```python
from build123d import *

# Parameters (mm, degrees)
F0_W      = 30.1625
F0_H      = 6.35
F1_DEPTH  = 26.9875
F3_DEPTH  = 6.351
F4_W      = 12.7
F4_H      = 6.35
F5_DEPTH  = 6.351
F6_W      = 6.35
F6_H      = 1.5875
F7_DEPTH  = 7.9375
F8_W      = 12.7
F8_H      = 6.35
F9_DEPTH  = 3
F10_W     = 12.7
F10_H     = 6.35
F11_DEPTH = 3
F12_W     = 6.35
F12_H     = 10.9375
F13_DEPTH = 8
F14_W     = 6.35
F14_H     = 9.35
F15_DEPTH = 8
F16_W     = 6.35
F16_H     = 17.6375
F17_DEPTH = 1
F18_W     = 6.35
F18_H     = 11.2875
F19_DEPTH = 1
F20_W     = 24.8125
F20_H     = 6.35
F21_DEPTH = 1
F22_W     = 31.1625
F22_H     = 6.35
F23_DEPTH = 1


with BuildPart() as f1:
    # F0 (on Top) → F1 (new body)
    with BuildSketch(Plane.XY):
        with Locations((3.826838, -2.493716)):
            Rectangle(F0_W, F0_H)
    extrude(amount=F1_DEPTH)

    # F2 (on face) → F3 (cut, through all)
    with BuildSketch(Plane.XZ.offset(5.668716)):
        Polygon((15.733088, 9.525), (15.733088, 23.8125), (-8.079412, 23.8125), (-8.079412, 1.5875), (-4.904412, 1.5875), (-4.904412, 0), (3.033088, 0), (3.033088, 9.525), align=None)
    extrude(amount=-F3_DEPTH, mode=Mode.SUBTRACT)

    # F4 (on face) → F5 (cut, through all)
    with BuildSketch(Plane.XZ.offset(5.668716)):
        with Locations((12.558088, 3.175)):
            Rectangle(F4_W, F4_H)
    extrude(amount=-F5_DEPTH, mode=Mode.SUBTRACT)

    # F6 (on face) → F7 (join)
    with BuildSketch(Plane.YZ.offset(-4.904412)):
        with Locations((-2.493716, 0.79375)):
            Rectangle(F6_W, F6_H)
    extrude(amount=F7_DEPTH)

    # F8 (on face) → F9 (join)
    with BuildSketch(Plane.XY.offset(9.525)):
        with Locations((9.383088, -2.493716)):
            Rectangle(F8_W, F8_H)
    extrude(amount=F9_DEPTH)

    # F10 (on face) → F11 (cut)
    with BuildSketch(Plane(origin=(0, 0, 6.35), x_dir=(1, 0, 0), z_dir=(0, 0, -1))):
        with Locations((12.558088, 2.493716)):
            Rectangle(F10_W, F10_H)
    extrude(amount=-F11_DEPTH, mode=Mode.SUBTRACT)

    # F12 (on face) → F13 (join)
    with BuildSketch(Plane(origin=(3.033088, 0, 0), x_dir=(0, -1, 0), z_dir=(-1, 0, 0))):
        with Locations((2.493716, 7.05625)):
            Rectangle(F12_W, F12_H)
    extrude(amount=F13_DEPTH)

    # F14 (on face) → F15 (cut)
    with BuildSketch(Plane.YZ.offset(6.208088)):
        with Locations((-2.493716, 4.675)):
            Rectangle(F14_W, F14_H)
    extrude(amount=-F15_DEPTH, mode=Mode.SUBTRACT)

    # F16 (on face) → F17 (join)
    with BuildSketch(Plane.YZ.offset(18.908088)):
        with Locations((-2.493716, 18.16875)):
            Rectangle(F16_W, F16_H)
    extrude(amount=F17_DEPTH)

    # F18 (on face) → F19 (cut)
    with BuildSketch(Plane(origin=(15.733088, 0, 0), x_dir=(0, -1, 0), z_dir=(-1, 0, 0))):
        with Locations((2.493716, 18.16875)):
            Rectangle(F18_W, F18_H)
    extrude(amount=-F19_DEPTH, mode=Mode.SUBTRACT)

    # F20 (on face) → F21 (cut)
    with BuildSketch(Plane(origin=(0, 0, 23.8125), x_dir=(1, 0, 0), z_dir=(0, 0, -1))):
        with Locations((4.326838, 2.493716)):
            Rectangle(F20_W, F20_H)
    extrude(amount=-F21_DEPTH, mode=Mode.SUBTRACT)

    # F22 (on face) → F23 (join)
    with BuildSketch(Plane.XY.offset(26.9875)):
        with Locations((4.326838, -2.493716)):
            Rectangle(F22_W, F22_H)
    extrude(amount=F23_DEPTH)


solid = f1.part
```
Geometry check sheet. Reference: the model listing, model coordinates, mm. A direction names the side the tool comes from. Give positions to 0.01 mm unless a question says otherwise; leave off trailing zeros. Loops run counter-clockwise (first coordinate to the right, second up) from the corner with the lowest first, then second, coordinate; pieces in that order, holes last. Notation, with made-up numbers: (-22, 54) - (6, 54) arc R15 ccw to (6, 59) - close; hole circle Ø4 at (-30.5, 9). An arc over 180 degrees is marked (long way). Use CSV: the item, a comma, the result in double quotes. Start each with the question number.
Q1. Go/stop test with flat-tipped pins: pin 1 Ø3 at (x, y) = (6.5, -3) entering from -Z; pin 2 Ø4 at (x, z) = (-6, 20.5) entering from +Y; pin 3 Ø3 at (y, z) = (-3.5, 3) entering from +X. Record where each tip stops, or that it passes through.
Q2. Release check for a two-part mould opening along X. For faces 4 (the face through (-1.792, -3, 5)), 5 (the face through (6, -2, 12.525)), 6 (the face through (1, 0.681, 11)) record: +X half, -X half, draft (parallel to the pull), parting line (faces both ways), or undercut.
Q3. Access from +Z, -Z, +X, -X, +Y, -Y to the whole of each face (thin tool, end or side, straight path). Record for faces 1 (the face through (19.908, -3, 19)), 2 (the face through (-8.079, -2, 13)), 3 (the face through (9, -3, 9.35)).
Q4. Scan lines: probe 1 along X at (y, z) = (-4.75, 14.75); probe 2 along X at (y, z) = (-2.5, 6); probe 3 along Z at (x, y) = (-2, -1.25) (1 decimal). Record each from-to range of solid material in increasing order. Write a range as from..to.
Q5. Section check A-A, the plane z = 9.75. Record the cut outline in (x, y).
Findings below:
1,pin 1,"stops at z = 9.35"
1,pin 2,"passes through"
1,pin 3,"stops at x = -1.79"
2,face 4,"+X half"
2,face 5,"undercut"
2,face 6,"draft"
3,face 1,"+Z, -Z, +X, +Y, -Y"
3,face 2,"+Y, -Y"
3,face 3,"-Z, +X, +Y, -Y"
4,probe 1,"x = -11.25..-8.08, 16.73..19.91"
4,probe 2,"x = -11.25..-8.08, -4.97..-1.79"
4,probe 3,"z = 0..12.5, 24.8..28"
5,outline,"(-11.25, -5.67) - (-8.08, -5.67) - (-8.08, 0.68) - (-11.25, 0.68) - close; (-4.97, -5.67) - (19.91, -5.67) - (19.91, 0.68) - (-4.97, 0.68) - close"
